Can you work these out from the model? Positions are in its coordinate system, mm. A direction names the side the tool comes from. Round coordinates to 2 decimals unless told otherwise and drop trailing zeros. Order: outer loops, then holes, each group sorted by start corner. A loop starts at its lowest first (then second) coordinate and runs counter-clockwise, first axis right, second up. Notation, with made-up numbers: M -23,32.5 L -5,32.5 A16 ccw -5,63.5 Z; hole C -21.75,-16.5 d8. An arc over 180 degrees is marked long. Answer as a JSON object with one key per item and string values. Group by question number.
```python
from build123d import *

# Parameters (mm, degrees)
F0_W      = 84.8816260695
F0_H      = 77.4099454284
F1_DEPTH  = 40.64
F2_DEPTH  = 38.1
F3_SIZE   = 5.08
F4_DEPTH  = 12.7
F5_W      = 93.0721817722
F5_H      = 115.5099454284
F6_DEPTH  = 25.4
F7_W      = 36.0550768673
F7_H      = 25.6806416437
F7_H_2    = 18.3557639778
F7_H_3    = 24.3065860122
F8_DEPTH  = 15.24
F9_W      = 38.0150713027
F9_H      = 24.3256706744
F9_H_2    = 25.5810311064
F9_W_2    = 38.3858084679
F9_H_3    = 18.5193228483
F10_DEPTH = 12.7
F11_R     = 5.08
F12_W     = 29.0874056518
F12_H     = 21.6887369752
F12_W_2   = 28.9331488311
F12_H_2   = 23.4388820827
F13_DEPTH = 25.4
F14_SIZE  = 15.24
F15_R     = 8.0063032483
F15_R_2   = 6.2284075283
F16_DEPTH = 2.54


with BuildPart() as f1:
    # F0 (on Right) → F1 (new body)
    with BuildSketch(Plane.YZ):
        with Locations((6.3857361674, -0.295586884)):
            Rectangle(F0_W, F0_H)
    extrude(amount=-F1_DEPTH)

    # F2 (add): a face of the model
    f2_faces = [f1.faces().sort_by_distance(p)[0] for p in [
        (-20.32, 6.3857361674, 38.4093858302),
    ]]
    extrude(f2_faces, amount=F2_DEPTH)

    # F3
    f3_edges = [f1.edges().sort_by_distance(p)[0] for p in [
        (0, 48.826549, 18.754413),
    ]]
    chamfer(f3_edges, length=F3_SIZE)

    # F4 (add): a face of the model
    f4_faces = [f1.faces().sort_by_distance(p)[0] for p in [
        (-2.54, 46.2865492022, 18.754413116),
    ]]
    extrude(f4_faces, amount=F4_DEPTH)

    # F5 (on face) → F6 (join)
    with BuildSketch(Plane(origin=(30.8535307222, 30.8535307222, 0), x_dir=(-0.7071067812, 0.7071067812, 0), z_dir=(0.7071067812, 0.7071067812, 0))):
        with Locations((-8.4184043949, 18.754413116)):
            Rectangle(F5_W, F5_H)
    extrude(amount=F6_DEPTH)

    # F7 (on face) → F8 (join)
    with BuildSketch(Plane.YZ):
        with Locations((-18.0275384337, 22.2555273212)):
            Rectangle(F7_W, F7_H)
        with Locations((-18.0275384337, 67.3315038413)):
            Rectangle(F7_W, F7_H_2)
        with Locations((-18.0275384337, -26.8472665921)):
            Rectangle(F7_W, F7_H_3)
    extrude(amount=F8_DEPTH)

    # F9 (on face) → F10 (join)
    with BuildSketch(Plane(origin=(30.8535307222, 30.8535307222, 0), x_dir=(0.7071067812, -0.7071067812, 0), z_dir=(-0.7071067812, -0.7071067812, 0))):
        with Locations((35.9469596297, -26.837724261)):
            Rectangle(F9_W, F9_H)
        with Locations((35.9469596297, 22.0283274539)):
            Rectangle(F9_W, F9_H_2)
        with Locations((35.761591047, 67.249724406)):
            Rectangle(F9_W_2, F9_H_3)
    extrude(amount=F10_DEPTH)

    # F11
    f11_edges = [f1.edges().sort_by_distance(p)[0] for p in [
        (15.24, -36.055077, 67.331504),
        (15.24, -18.027538, 76.509386),
        (15.24, 0, 67.331504),
        (15.24, -18.027538, 35.095848),
        (15.24, -36.055077, 22.255527),
        (15.24, -18.027538, 9.415206),
        (15.24, 0, 22.255527),
        (15.24, -36.055077, -26.847267),
        (15.24, -18.027538, -39.00056),
        (15.24, 0, -26.847267),
        (15.24, -18.027538, -14.693974),
        (60.731971, -16.985422, 67.249724),
        (47.160538, -3.413989, 76.509386),
        (33.589105, 10.157444, 67.249724),
        (47.160538, -3.413989, 57.990063),
        (60.731971, -16.985422, 22.028327),
        (47.291614, -3.545064, 34.818843),
        (33.851256, 9.895293, 22.028327),
        (47.291614, -3.545064, 9.237812),
        (33.851256, 9.895293, -26.837724),
        (47.291614, -3.545064, -39.00056),
        (60.731971, -16.985422, -26.837724),
        (47.291614, -3.545064, -14.674889),
    ]]
    fillet(f11_edges, radius=F11_R)

    # F12 (on face) → F13 (join)
    with BuildSketch(Plane(origin=(48.8140429643, 48.8140429643, 0), x_dir=(-0.7071067812, 0.7071067812, 0), z_dir=(0.7071067812, 0.7071067812, 0))):
        with Locations((-40.4107924551, -10.8443684876)):
            Rectangle(F12_W, F12_H)
        with Locations((-40.4879208654, 38.8789121062)):
            Rectangle(F12_W_2, F12_H_2)
    extrude(amount=F13_DEPTH)

    # F14
    f14_edges = [f1.edges().sort_by_distance(p)[0] for p in [
        (105.633251, 27.915859, 38.878912),
        (105.633251, 27.915859, -10.844368),
    ]]
    chamfer(f14_edges, length=F14_SIZE)

    # F15 (on face) → F16 (join)
    with BuildSketch(Plane.YZ.offset(94.856944131)):
        with Locations((28.4049902111, 37.9507169127)):
            Circle(F15_R)
        with Locations((28.1626116484, -12.1466107666)):
            Circle(F15_R_2)
    extrude(amount=F16_DEPTH)


solid = f1.part
```
1) I need wall thicknesses on line 1 along Z through (x, y) = (63.5, -2); line 2 along X through (y, z) = (-19, 61.5); line 3 along X through (y, z) = (-9, 3). Which ranges of each line are inside material? Lowest first, please.
2) We'd pull the mould along Z, two halves only. Please class faces 6 (the face through (-7, 19, -39.001)), 7 (the face through (13.71, -34.61, 67.46)), 8 (the face through (48.56, -2.653, 10.686)): +Z half, -Z half, draft (parallel to the pull), parting line (faces both ways), or undercut.
3) If we section it at D-D on z = 7.5: Write out the boundary of the cut face in (x, y).
4) If we section it at C-C on x = 40.5: Count the separate pieces of the cut face and the enclosed holes in it, plus the area to 3 significant figures.
5) For pin 1 (4 mm diameter, centred on y = -20.5, z = -26.5, fed in from +X); pin 2 (1 mm diameter, centred on x = 76, z = 36, fed in from +Y); pin 3 (3 mm diameter, centred on x = 3.5, z = 70, fed in from +Y), each with a flat end and sliding along its axis, tell me the tip position at first contact or that it passes through.
6) If we section it at A-A on y = 51: Write out the boundary of the cut face in (x, z).
7) Which directions (+Z, -Z, +X, -X, +Y, -Y) give clear straight access to the entire face, cutting with the end or side of a thin tool? Please do faces 1 (the face through (13.791, -1.528, -26.677)), 2 (the face through (84, 31, 0)), 3 (the face through (40.175, 16.219, 21.849)), 4 (the face through (48.56, -2.65, 33.37)), 5 (the face through (15.24, -18, 65)).
8) If we section it at B-B on z = 66: Write out the boundary of the cut face in (x, y).
Findings:
{
 "1": {"line 1": "z = -39 to -14.67, 9.24 to 34.82, 57.99 to 76.51", "line 2": "x = -40.64 to 15.24", "line 3": "x = -40.64 to 0"},
 "2": {"face 6": "-Z half", "face 7": "draft", "face 8": "undercut"},
 "3": {"outline": "M -40.64,-36.06 L 0,-36.06 L 0,43.75 L 8.98,52.73 L 69.71,-8.01 L 87.67,9.96 L 21.86,75.77 L -5.08,48.83 L -40.64,48.83 Z"},
 "4": {"separate pieces": "4", "enclosed holes": "0", "area": "5,020 mm^2"},
 "5": {"pin 1": "stops at x = 15.24", "pin 2": "stops at y = 39.7", "pin 3": "stops at y = 58.91"},
 "6": {"outline": "M -2.91,-39 L 7.25,-39 L 7.25,76.51 L -2.91,76.51 Z; M 10.71,-39 L 46.63,-39 L 46.63,76.51 L 10.71,76.51 Z"},
 "7": {"face 1": "+Z, -Z", "face 2": "+X, +Y", "face 3": "-Z", "face 4": "-Y", "face 5": "+Z, -Z, -Y"},
 "8": {"outline": "M -40.64,-36.06 L 10.16,-36.06 A5.08 ccw 15.24,-30.98 L 15.24,-5.08 A5.08 ccw 10.16,0 L 0,0 L 0,43.75 L 8.98,52.73 L 42.57,19.14 L 37.18,13.75 A5.08 ccw 37.18,6.57 L 57.14,-13.39 A5.08 ccw 64.32,-13.39 L 87.67,9.96 L 21.86,75.77 L -5.08,48.83 L -40.64,48.83 Z"}
}
